from build123d import *

# Parameters (mm, degrees)
F0_W       = 98.3872264624
F0_H       = 78.1223997474
F1_DEPTH   = 2.54
F2_W       = 10.5729550123
F2_H       = 78.1223997474
F1_FACE1_W = 98.3872264624
F1_FACE1_H = 78.1223997474
F3_DEPTH   = 6.35
F5_W       = 10.6261968613
F5_H       = 76.7848268151
F6_DEPTH   = 6.35


with BuildPart() as f1:
    # F0 (on Top) → F1 (new body)
    with BuildSketch(Plane.XY):
        with Locations((2.7900859714, 3.524325788)):
            Rectangle(F0_W, F0_H)
    extrude(amount=F1_DEPTH)

    # F2 (on face) + F1_face1 (on face) → F3 (join)
    with BuildSketch(Plane.XY.offset(2.54)):
        with Locations((-32.5999483466, 3.524325788)):
            Rectangle(F2_W, F2_H)
    with BuildSketch(Plane(origin=(2.7900859714, 3.524325788, 0), x_dir=(1, 0, 0), z_dir=(0, 0, -1))):
        Rectangle(F1_FACE1_W, F1_FACE1_H)
    extrude(amount=F3_DEPTH, dir=(0, 0, 1))

    # F5 (on face) → F6 (join)
    with BuildSketch(Plane(origin=(0, 0, 0), x_dir=(1, 0, 0), z_dir=(0, 0, -1))):
        with Locations((-32.4897877872, -4.1658058763)):
            Rectangle(F5_W, F5_H)
    extrude(amount=F6_DEPTH)


solid = f1.part
Geometry: final body of the model. Coordinates: model frame, mm. A direction names the side the tool comes from. Coordinates: 2 decimals unless noted, no trailing zeros. Loops run counter-clockwise (first coordinate to the right, second up) from the corner with the lowest first, then second, coordinate; pieces in that order, holes last. Notation, with made-up numbers: (-25.5, -24.5) - (29.5, -24.5) arc R6 ccw to (29.5, -16.5) - close; hole circle Ø1 at (21.25, -11). An arc over 180 degrees is marked (long way). Put each result on its own line as item: value. Start each with the question number.
Q1. Cut plane B-B, the plane z = -4.75. Return loops of the section in (x, y), and give its area (3 significant figures).
Q2. Cut plane A-A, the plane y = 6. Return loops of the section in (x, z), and give its area (3 significant figures).
Q3. Pin query (flat end, axial travel): pin 1 Ø1.9 at (y, z) = (0, -3) entering from +X; pin 2 Ø1.9 at (x, z) = (-33, -2.5) entering from +Y; pin 3 Ø1 at (y, z) = (27.5, 7) entering from +X. Return the tip coordinate at first contact, or that it passes through.
Q4. Set-up query: faces 1 (the flat face through (-37.886, 3, 8)), 2 (the flat face through (-33, -34.227, -3)), 3 (the flat face through (-27.177, 5, -3)). Return all of +Z, -Z, +X, -X, +Y, -Y with unobstructed straight access to the full face (end or side cutting, diameter ignored); none if empty.
Q5. Line query: line 1 (Z direction, x = -12.5, y = -9.5); line 2 (X direction, y = 28.5, z = -3.75); line 3 (X direction, y = -12.5, z = 7.5). Output: solid intervals per line, ascending.
Q6. Cut plane C-C, the plane x = -7. Return loops of the section in (y, z).
Filled sheet:
1. outline: (-37.8, -34.23) - (-27.18, -34.23) - (-27.18, 42.56) - (-37.8, 42.56) - close
1. area: 816 mm²
2. outline: (-46.4, 0) - (-37.8, 0) - (-37.8, -6.35) - (-27.18, -6.35) - (-27.18, 0) - (51.98, 0) - (51.98, 6.35) - (-27.31, 6.35) - (-27.31, 8.89) - (-37.89, 8.89) - (-37.89, 6.35) - (-46.4, 6.35) - close
2. area: 719 mm²
3. pin 1: x = -27.18
3. pin 2: y = 42.56
3. pin 3: x = -27.31
4. face 1: +Z, -X, +Y, -Y
4. face 2: -Z, +X, -X, -Y
4. face 3: -Z, +X, +Y, -Y
5. line 1: 0 to 6.35
5. line 2: -37.8 to -27.18
5. line 3: -37.89 to -27.31
6. outline: (-35.54, 0) - (42.59, 0) - (42.59, 6.35) - (-35.54, 6.35) - close
